Design review of the part built by this model. Coordinates are the model's own, in mm. Face numbers are marked on the shaded views. A direction names the side the tool comes from. Give positions to 0.01 mm unless a question says otherwise; leave off trailing zeros. Write each loop counter-clockwise with the first axis right and the second up, starting at its lowest first coordinate (ties: lowest second). Pieces come first, ordered by that corner, then holes. Notation, with made-up numbers: M 46.25,26 L 99.25,26 A24 ccw 99.25,63 Z; hole C -5,6.25 d9. An arc over 180 degrees is marked long. Answer in a Markdown table with one row per item.
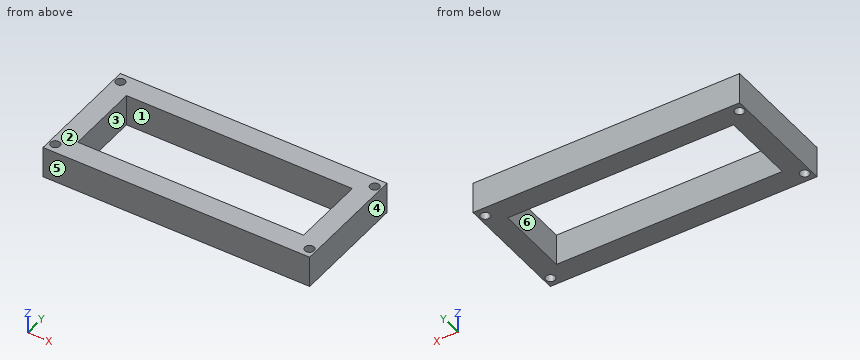
```python
from build123d import *

# Parameters (mm, degrees)
SKETCH1_W           = 86.199999926
SKETCH1_H           = 38.1
SKETCH1_W_2         = 73
SKETCH1_H_2         = 24
BOSS_EXTRUDE1_DEPTH = 10.16
SKETCH2_R           = 1.5
CUT_EXTRUDE1_DEPTH  = 10.16


with BuildPart() as part:
    # Sketch1 → Boss-Extrude1 (new body)
    with BuildSketch(Plane.XY):
        Rectangle(SKETCH1_W, SKETCH1_H)
        Rectangle(SKETCH1_W_2, SKETCH1_H_2, mode=Mode.SUBTRACT)
    extrude(amount=BOSS_EXTRUDE1_DEPTH)

    # Sketch2 → Cut-Extrude1 (cut)
    with BuildSketch(Plane.XY.offset(10.16)):
        with Locations((41.099999963, 16.05)):
            Circle(SKETCH2_R)
        with Locations(Location((-41.099999963, 16.05, 0), (0, 0, 180))):
            Circle(SKETCH2_R)
        with Locations((-41.099999963, -16.05)):
            Circle(SKETCH2_R)
        with Locations(Location((41.099999963, -16.05, 0), (0, 0, 180))):
            Circle(SKETCH2_R)
    extrude(amount=-CUT_EXTRUDE1_DEPTH, mode=Mode.SUBTRACT)


solid = part.part
```
1) The part is to be moulded in two halves that separate along X. For the marked faces 1, 2, 3 and 4, say which applies: released by +X, released by -X, zero draft, split by the parting line, or undercut.
Geometry says:
| item | result |
|---|---|
| face 1 | undercut |
| face 2 | zero draft |
| face 3 | undercut |
| face 4 | released by +X |
2) Add section D-D (z = 7). Write out the cut boundary in (x, y), and give its area (3 significant figures).
Geometry says:
| item | result |
|---|---|
| outline | M -43.1,-19.05 L 43.1,-19.05 L 43.1,19.05 L -43.1,19.05 Z; hole C -41.1,-16.05 d3; hole C -41.1,16.05 d3; hole M -36.5,-12 L 36.5,-12 L 36.5,12 L -36.5,12 Z; hole C 41.1,-16.05 d3; hole C 41.1,16.05 d3 |
| area | 1,500 mm^2 |
3) Add section B-B (x = 30). Write out the cut boundary in (y, z).
Geometry says:
| item | result |
|---|---|
| outline | M -19.05,0 L -12,0 L -12,10.16 L -19.05,10.16 Z; M 12,0 L 19.05,0 L 19.05,10.16 L 12,10.16 Z |
4) Add section A-A (y = -8). Write out the cut boundary in (x, z).
Geometry says:
| item | result |
|---|---|
| outline | M -43.1,0 L -36.5,0 L -36.5,10.16 L -43.1,10.16 Z; M 36.5,0 L 43.1,0 L 43.1,10.16 L 36.5,10.16 Z |
5) To check wall thickness, follow probe 1 along X at (y, z) = (16, 5.5); probe 2 along Y at (x, z) = (-41.1, 5.25); probe 3 along X at (y, z) = (4.5, 2.5). State the ranges of each line that lie inside material, in increasing order. Write a range as [from, to].
Geometry says:
| item | result |
|---|---|
| probe 1 | [-43.1, -42.6], [-39.6, 39.6], [42.6, 43.1] |
| probe 2 | [-19.05, -17.55], [-14.55, 14.55], [17.55, 19.05] |
| probe 3 | [-43.1, -36.5], [36.5, 43.1] |
6) Add section C-C (x = 41.1). Write out the cut boundary in (y, z).
Geometry says:
| item | result |
|---|---|
| outline | M -19.05,0 L -17.55,0 L -17.55,10.16 L -19.05,10.16 Z; M -14.55,0 L 14.55,0 L 14.55,10.16 L -14.55,10.16 Z; M 17.55,0 L 19.05,0 L 19.05,10.16 L 17.55,10.16 Z |
7) Insertion check: P1, Ø2.5, axis at x = 41.1, y = -16.05, coming from the -Z side. The pin has a flat end and moves straight along its axis. Give the tip position at first contact, or say it passes through.
Geometry says:
| item | result |
|---|---|
| P1 | through |
8) For the marked faces 5 and 6, list the 3-axis set-ups (+Z, -Z, +X, -X, +Y, -Y) from which the entire face can be reached by the end or side of a thin tool; tool diameter is ignored.
Geometry says:
| item | result |
|---|---|
| face 5 | +Z, -Z, +X, -X, -Y |
| face 6 | +Z, -Z |
